from build123d import *

# Parameters (mm, degrees)
SKETCH1_W = 550
SKETCH1_H = 1.6
SKETCH2_W = 9.6
SKETCH2_H = 8.524943062


with BuildPart() as part:
    # Sketch1 → Revolve1 (revolve)
    with BuildSketch(Plane.XY, mode=Mode.PRIVATE) as revolve1_sk:
        with Locations((82.249266675, 26.2)):
            Rectangle(SKETCH1_W, SKETCH1_H)
    revolve(revolve1_sk.sketch.rotate(Axis((-404.790100073, 0, 0), (1, 0, 0)), 90), axis=Axis((-404.790100073, 0, 0), (1, 0, 0)))

    # Sketch2 → Revolve2 (revolve)
    with BuildSketch(Plane.XY, mode=Mode.PRIVATE) as revolve2_sk:
        with Locations((362.049266675, 24.237528469)):
            Rectangle(SKETCH2_W, SKETCH2_H)
        Polygon((-176.750733325, 27), (-176.750733325, 14.5), (-202.260733325, 14.5), (-202.260733325, 0), (-204.250733325, 0), (-204.250733325, 11), (-211.750733325, 11), (-211.750733325, 19), (-195.850733325, 19), (-195.850733325, 27), align=None)
    revolve(revolve2_sk.sketch.rotate(Axis((-209.882463346, 0, 0), (1, 0, 0)), 90), axis=Axis((-209.882463346, 0, 0), (1, 0, 0)))


solid = part.part
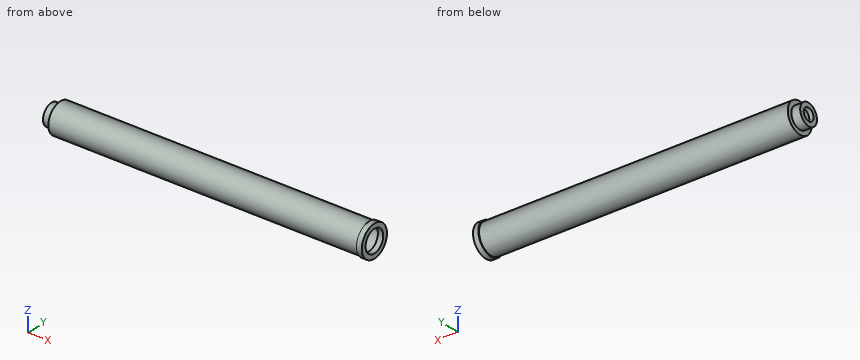
Design review of the part built by this model. Coordinates are the model's own, in mm. Give positions to 0.01 mm unless a question says otherwise; leave off trailing zeros. Loops run counter-clockwise (first coordinate to the right, second up) from the corner with the lowest first, then second, coordinate; pieces in that order, holes last. Notation, with made-up numbers: (37, 85.5) -> (63, 85.5) arc R14 ccw to (63, 95.5) -> close; hole circle Ø10 at (76.5, 5.25). An arc over 180 degrees is marked (long way). One line per question, with ' | ' between items. Start each with the question number.
(1) We need section B-B (x = 253). State the section outline as (y, z) points.
(2) Insertion check: P1, Ø13, axis at y = 0, z = 0, coming from the +X side; P2, Ø2, axis at x = 23, z = 3.5, coming from the -Y side; P3, Ø8, axis at x = 205.5, y = 11, coming from the -Z side. Each pin has a flat end and moves straight along its axis. Give the tip position at first contact, or say it passes through.
(3) We need section A-A (z = 0). State the section outline as (x, y) points.
(4) For line 1 (Y direction, x = -193, z = 0); line 2 (Y direction, x = -206.5, z = 0); line 3 (X direction, y = -6.5, z = 23.5), list the stretches that pass through material, from the lowest coordinate up.
The answers:
1) outline: circle Ø54 at (0, 0); hole circle Ø50.8 at (0, 0)
2) P1: stops at x = -202.26 | P2: stops at y = -26.88 | P3: stops at z = -26.08
3) outline: (-211.75, -19) -> (-195.85, -19) -> (-195.85, -27) -> (357.25, -27) -> (357.25, -28.5) -> (366.85, -28.5) -> (366.85, -19.98) -> (357.25, -19.98) -> (357.25, -25.4) -> (-176.75, -25.4) -> (-176.75, -14.5) -> (-202.26, -14.5) -> (-202.26, 14.5) -> (-176.75, 14.5) -> (-176.75, 25.4) -> (357.25, 25.4) -> (357.25, 19.98) -> (366.85, 19.98) -> (366.85, 28.5) -> (357.25, 28.5) -> (357.25, 27) -> (-195.85, 27) -> (-195.85, 19) -> (-211.75, 19) -> (-211.75, 11) -> (-204.25, 11) -> (-204.25, -11) -> (-211.75, -11) -> close
4) line 1: y = -27 to -14.5, 14.5 to 27 | line 2: y = -19 to -11, 11 to 19 | line 3: x = -195.85 to -176.75, 357.25 to 366.85
